The listing builds one solid part. Answer for the finished solid, in the listing's coordinates (mm). A direction names the side the tool comes from. Round coordinates to 2 decimals unless told otherwise and drop trailing zeros. Write each loop counter-clockwise with the first axis right and the second up, starting at its lowest first coordinate (ties: lowest second). Pieces come first, ordered by that corner, then holes.
(1) A cutting plane is placed at C-C, the plane z = -42.5. Give the vertices of the cut face in (x, y), and give its area (3 significant figures).
(2) Find the intervals of material crossed by probe 1 along Y at (x, z) = (6.75, -10); probe 2 along Y at (x, z) = (30, -44); probe 3 along Z at (x, y) = (11.5, 39.5), in increasing order.
(3) For faces 5 (the face through (26, 8, -30)), 6 (the face through (5, 20, -25)), 7 (the face through (45, 10, -40)), 8 (the face through (25, 15, -35)), determine the directions among +Z, -Z, +X, -X, +Y, -Y from which every point of the face is accessible in a straight line to the end or side of a thin tool.
(4) Each of these flat-tipped pins is pushed along its axis until it touches: pin 1 Ø8 at (x, y) = (23, 35) entering from +Z; pin 2 Ø2 at (x, z) = (33, -35) entering from -Y; pin 3 Ø5 at (y, z) = (31, -45) entering from +X; pin 4 Ø10 at (y, z) = (14.5, -12) entering from +X. Where does it stop, or does it pass through?
(5) A cutting plane is placed at D-D, the plane x = 31. Give the vertices of the cut face in (y, z).
(6) A cutting plane is placed at B-B, the plane y = 30. Give the vertices of the cut face in (x, z).
(7) The mould has two halves that part along X. Classify faces 1 (the face through (25, 30, -45)), 2 (the face through (5.07, 17.15, -3.01)), 3 (the face through (0, 19, -31)), 4 (the face through (40, 25, -45)): +X half, -X half, draft (parallel to the pull), parting line (faces both ways), or undercut.
(8) A cutting plane is placed at A-A, the plane z = -14. Give the vertices of the cut face in (x, y), and give its area (3 significant figures).
Autodesk Inventor part; units mm, degrees
ref_plane "YZ Plane" through (0, 0, 0) normal (1, 0, 0) x (0, 1, 0)
ref_plane "XZ Plane" through (0, 0, 0) normal (0, 1, 0) x (-1, 0, 0)
ref_plane "XY Plane" through (0, 0, 0) normal (0, 0, 1) x (1, 0, 0)
sketch "草圖1" plane through (0, 0, 0) normal (0, 1, 0) x (-1, 0, 0)
  line L0 (0, 0) -> (-10, 0)
  line L1 (-10, 0) -> (-10, -50)
  line L2 (-10, -50) -> (0, -50)
  line L3 (0, -50) -> (0, 0)
  line L4 (-10, -50) -> (-50, -50)
  line L5 (-50, -50) -> (-50, -30)
  line L6 (-50, -30) -> (-10, -30)
  line L7 (-10, -30) -> (-10, -50)
  dimension "d0" = 20
  dimension "d1" = 10
  dimension "d2" = 50
  dimension "d3" = 40
extrude "擠出1" add sketch "草圖1" along normal blind 20
sketch "草圖2" plane through (10, 0, -30) normal (0, 0, 1) x (1, 0, 0)
  line L0 (0, 0) -> (0, 20)
  line L1 (0, 20) -> (30, 10)
  line L2 (30, 10) -> (42.5125, 10)
  line L3 (0, 0) -> (40, 0)
  line L4 (0, 20) -> (41.4864, 29.1876)
  line L5 (41.4864, 29.1876) -> (42.5125, 10)
  point P0 (-10, 0)
  dimension "d6" = 10
  dimension "d7" = 30
extrude "擠出2" cut sketch "草圖2" against normal through all
sketch "草圖3" plane through (50, 0, -50) normal (0, 0, -1) x (-1, 0, 0)
  line L0 (50, 0) -> (10, 0)
  line L1 (10, 0) -> (10, 50)
  line L2 (10, 50) -> (50, 50)
  line L3 (50, 50) -> (50, 0)
  dimension "d12" = 40
  dimension "d13" = 50
extrude "擠出3" add sketch "草圖3" against normal blind 10
chamfer "倒角1" distance 10 distance2 20 1 edges at (40, 50, -45) measured on face at (40, 23.3333, -46.6667)
fillet "圓角1" radius 10 1 edges at (5, 20, 0)
sketch "草圖4" plane through (10, 0, 0) normal (1, 0, 0) x (0, 0, -1)
  circle A0 centre (10, 10) radius 5
  line L0 (0, 0) -> (30, 0)
  line L1 (0, 0) -> (0, 10)
  dimension "d20" = 10
  dimension "d21" = 10
  dimension "d22" = 10
extrude "擠出4" cut sketch "草圖4" against normal blind 10
sketch "草圖5" plane through (50, 0, -40) normal (0, 0, 1) x (1, 0, 0)
  circle A0 centre (-20, 30) radius 5
  line L0 (-10, 10) -> (-10, 40)
  point P0 (-50, 0)
  dimension "d25" = 10
  dimension "d26" = 10
  dimension "d27" = 10
extrude "擠出5" cut sketch "草圖5" against normal blind 10
properties part number "30"
Solutions:
1. outline: (0, 0) - (50, 0) - (50, 10) - (40, 10) - (40, 40) - (20, 50) - (0, 50) - close; hole circle Ø10 at (30, 30)
1. area: 1,920 mm2
2. probe 1: y = 0 to 5, 15 to 20
2. probe 2: y = 0 to 25, 35 to 45
2. probe 3: z = -50 to -40
3. face 5: +Z, +X, +Y, -Y
3. face 6: +Z, +X, -X, +Y
3. face 7: +Z, -Z, +X, +Y
3. face 8: +Z, +X, +Y
4. pin 1: stops at z = -40
4. pin 2: stops at y = 0
4. pin 3: stops at x = 40
4. pin 4: stops at x = 10
5. outline: (0, -50) - (25.1, -50) - (25.1, -40) - (13, -40) - (13, -30) - (0, -30) - close; (34.9, -50) - (44.5, -50) - (44.5, -40) - (34.9, -40) - close
6. outline: (0, -50) - (25, -50) - (25, -40) - (0, -40) - close; (35, -50) - (40, -50) - (40, -40) - (35, -40) - close
7. face 1: undercut
7. face 2: draft
7. face 3: -X half
7. face 4: +X half
8. outline: (0, 0) - (10, 0) - (10, 7) - (0, 7) - close; (0, 13) - (10, 13) - (10, 20) - (0, 20) - close
8. area: 140 mm2
